Geometry check sheet. Reference: the model listing, model coordinates, mm. A direction names the side the tool comes from. Round coordinates to 2 decimals unless told otherwise and drop trailing zeros. Order: outer loops, then holes, each group sorted by start corner. A loop starts at its lowest first (then second) coordinate and runs counter-clockwise, first axis right, second up. Notation, with made-up numbers: M 81.25,81 L 101.25,81 A23 cw 101.25,90 Z; hole C -20.5,35 d1. An arc over 180 degrees is marked long. Answer as a JSON object with one key per item and string values. Group by question number.
```python
from build123d import *
from build123d.topology import SkipClean

# Parameters (mm, degrees)
EXTRUDE_1_DEPTH     = 12.1
SKETCH_2_W          = 2.5
SKETCH_2_H          = 6
CUT_EXTRUDE_1_DEPTH = 5
SKETCH_3_R          = 2.5
CUT_EXTRUDE_2_DEPTH = 4
CUT_EXTRUDE_3_DEPTH = 3
SKETCH_5_W          = 6
SKETCH_5_H          = 12
CUT_EXTRUDE_4_DEPTH = 5
FILLET_1_R          = 3
SKETCH_6_R          = 5
SKETCH_6_R_2        = 1.65
CUT_EXTRUDE_5_DEPTH = 5
SKETCH_7_W          = 8
SKETCH_7_H          = 2.5
EXTRUDE_2_DEPTH     = 27
SKETCH_8_R          = 2.1
CUT_EXTRUDE_6_DEPTH = 30
CHAMFER_1_SIZE      = 2
CUT_EXTRUDE_7_DEPTH = 2


with BuildPart() as part:
    # Эскиз1 → Вытянуть1 (new body)
    with BuildSketch(Plane.XY):
        Polygon((0, -23), (0, 18), (-18, 18), (-32.3, 12.413885007), (-32.3, 2.413885007), (-25, -23), align=None)
    extrude(amount=EXTRUDE_1_DEPTH)

    # Эскиз2 → Вырез-Вытянуть1 (cut)
    with BuildSketch(Plane(origin=(0, 18, 0), x_dir=(1, 0, 0), z_dir=(0, 1, 0))):
        with Locations((-4.25, -6.05)):
            Rectangle(SKETCH_2_W, SKETCH_2_H)
    extrude(amount=-CUT_EXTRUDE_1_DEPTH, mode=Mode.SUBTRACT)

    # Эскиз3 → Вырез-Вытянуть2 (cut)
    with BuildSketch(Plane(origin=(-8.483646071, 21.717443871, 0), x_dir=(0.9314534311844429, 0.3638605578167664, 0), z_dir=(-0.3638605578167664, 0.931453431184443, 0))):
        with Locations(Location((-18.036153415, -6.05, 0), (0, 0, 180))):
            Circle(SKETCH_3_R)
    extrude(amount=-CUT_EXTRUDE_2_DEPTH, mode=Mode.SUBTRACT)

    # Эскиз4 → Вырез-Вытянуть3 (cut)
    with SkipClean():  # the faces are left unmerged after this step: merging them gives an invalid solid
        with BuildSketch(Plane(origin=(-7.028203839, 17.991630147, 0), x_dir=(0.9314534311844429, 0.3638605578167665, 0), z_dir=(-0.36386055781676646, 0.9314534311844428, 0))):
            with BuildLine():
                Line((-20.093115316, -7.470882731), (-16.615270683, -3.993038099))
                ThreePointArc((-16.615270683, -3.993038099), (-16.268386462, -4.282233047), (-15.979191513, -4.629117269))
                Line((-15.979191513, -4.629117269), (-19.457036146, -8.106961901))
                ThreePointArc((-19.457036146, -8.106961901), (-19.803920367, -7.817766953), (-20.093115316, -7.470882731))
            make_face()
        extrude(amount=-CUT_EXTRUDE_3_DEPTH, mode=Mode.SUBTRACT)

    # Эскиз5 → Вырез-Вытянуть4 (cut)
    with SkipClean():  # the faces are left unmerged after this step: merging them gives an invalid solid
        with BuildSketch(Plane(origin=(-29.1975513, -8.386837527, 0), x_dir=(0, 0, 1), z_dir=(-0.9611344752582023, -0.27608064124480053, 0))):
            with Locations((6.05, -1.983302044)):
                Rectangle(SKETCH_5_W, SKETCH_5_H)
        extrude(amount=-CUT_EXTRUDE_4_DEPTH, mode=Mode.SUBTRACT)

    # Скругление1
    fillet_1_edges = [part.edges().sort_by_distance(p)[0] for p in [
        (-32.3, 12.413885007, 6.05),
        (-18, 18, 6.05),
        (-25, -23, 6.05),
        (-32.3, 2.413885007, 6.05),
    ]]
    fillet(fillet_1_edges, radius=FILLET_1_R)

    # Эскиз6 → Вырез-Вытянуть5 (cut)
    with SkipClean():  # the faces are left unmerged after this step: merging them gives an invalid solid
        with BuildSketch(Plane(origin=(0, 0, 0), x_dir=(0, 0, -1), z_dir=(1, 0, 0))):
            with Locations(Location((-6.05, 0, 0), (0, 0, 90))):
                Circle(SKETCH_6_R)
            with Locations(Location((-6.05, 10, 0), (0, 0, 90))):
                Circle(SKETCH_6_R_2)
        extrude(amount=-CUT_EXTRUDE_5_DEPTH, mode=Mode.SUBTRACT)

    # Эскиз7 → Вытянуть2 (add)
    with SkipClean():  # the faces are left unmerged after this step: merging them gives an invalid solid
        with BuildSketch(Plane(origin=(-5, 0, 0), x_dir=(0, 0, -1), z_dir=(1, 0, 0))):
            with Locations((-6.05, 0)):
                Rectangle(SKETCH_7_W, SKETCH_7_H)
        extrude(amount=EXTRUDE_2_DEPTH)

    # Эскиз8 → Вырез-Вытянуть6 (cut)
    with SkipClean():  # the faces are left unmerged after this step: merging them gives an invalid solid
        with BuildSketch(Plane(origin=(0, 1.25, 0), x_dir=(1, 0, 0), z_dir=(0, 1, 0))):
            with Locations(Location((15.6, -6.05, 0), (0, 0, 180))):
                Circle(SKETCH_8_R)
        extrude(amount=-CUT_EXTRUDE_6_DEPTH, mode=Mode.SUBTRACT)

    # Фаска1
    chamfer_1_edges = [part.edges().sort_by_distance(p)[0] for p in [
        (22, 0, 10.05),
        (22, 0, 2.05),
    ]]
    chamfer(chamfer_1_edges, length=CHAMFER_1_SIZE)

    # Эскиз9 → Вырез-Вытянуть7 (cut)
    with SkipClean():  # the faces are left unmerged after this step: merging them gives an invalid solid
        with BuildSketch(Plane(origin=(0, 0, 0), x_dir=(0, 0, -1), z_dir=(1, 0, 0))):
            with BuildLine():
                Line((-11.05, -23), (-1.05, -23))
                Line((-1.05, -23), (-1.05, 0))
                ThreePointArc((-1.05, 0), (-6.05, -5), (-11.05, 0))
                Line((-11.05, 0), (-11.05, -23))
            make_face()
        extrude(amount=-CUT_EXTRUDE_7_DEPTH, mode=Mode.SUBTRACT)


solid = part.part
```
1) Thickness scan on line 1 along Z through (x, y) = (-1.3, 0); line 2 along Z through (x, y) = (-1.1, 10); line 3 along Y through (x, z) = (2, 2.5). Record the ranges inside material, lowest first. Write a range as [from, to].
2) Sectioned sample at A-A (x = 15.6). Record the boundary of the cut face in (y, z), then the cut area to 3 significant figures.
3) Set-up check for faces 1 (the cylindrical face through (-2.46, 10.89, 7.44)), 2 (the flat face through (-24.62, -15.38, 6.01)), 3 (the flat face through (-1, -12, 1.05)), 4 (the flat face through (-4, 16, 9.05)): record each of +Z, -Z, +X, -X, +Y, -Y from which the full face is reachable in a straight line by a thin tool's end or side.
4) Go/stop test with flat-tipped pins: P1, Ø0.8, axis at x = 10.5, y = 0, coming from the -Z side; P2, Ø5.5, axis at y = 16, z = 6, coming from the +X side; P3, Ø4, axis at y = -11.5, z = 4.5, coming from the +X side; P4, Ø4, axis at x = 15.6, z = 6.05, coming from the +Y side. Record where each tip stops, or that it passes through.
5) Sectioned sample at B-B (y = -11). Record the boundary of the cut face in (x, z).
6) Release check for a two-part mould opening along X. For faces 5 (the flat face through (0, 6, 6)), 6 (the flat face through (-12, -23, 6)), 7 (the cylindrical face through (-17.98, 17.95, 6.13)), 8 (the flat face through (-4, 16, 3.05)) record: +X half, -X half, draft (parallel to the pull), parting line (faces both ways), or undercut.
7) Sectioned sample at C-C (x = 9). Record the boundary of the cut face in (y, z).
Final values:
{
 "1": {"line 1": "z = [0, 1.05], [2.05, 10.05], [11.05, 12.1]", "line 2": "z = [0, 4.4], [7.7, 12.1]", "line 3": "y = [-1.25, 1.25]"},
 "2": {"outline": "M -1.25,2.05 L 1.25,2.05 L 1.25,3.95 L -1.25,3.95 Z; M -1.25,8.15 L 1.25,8.15 L 1.25,10.05 L -1.25,10.05 Z", "area": "9.50 mm^2"},
 "3": {"face 1": "+X", "face 2": "-X", "face 3": "+X, -Y", "face 4": "+Y"},
 "4": {"P1": "stops at z = 2.05", "P2": "stops at x = 0", "P3": "stops at x = -2", "P4": "passes through"},
 "5": {"outline": "M -28.45,0 L 0,0 L 0,1.05 L -2,1.05 L -2,11.05 L 0,11.05 L 0,12.1 L -28.45,12.1 L -28.45,9.05 L -23.24,9.05 L -23.24,3.05 L -28.45,3.05 Z"},
 "6": {"face 5": "+X half", "face 6": "draft", "face 7": "-X half", "face 8": "undercut"},
 "7": {"outline": "M -1.25,2.05 L 1.25,2.05 L 1.25,10.05 L -1.25,10.05 Z"}
}
